from build123d import *

# Parameters (mm, degrees)
SKETCH_1_R          = 15
SKETCH_1_R_2        = 4.4
SKETCH_1_R_3        = 1.45
EXTRUDE_1_DEPTH     = 21
SKETCH_2_R          = 7.7
CUT_EXTRUDE_1_DEPTH = 4
SKETCH_3_R          = 11.25
CUT_EXTRUDE_2_DEPTH = 9.5
SKETCH_4_R          = 0.9
CUT_EXTRUDE_3_DEPTH = 4
SKETCH_5_W          = 6.5
SKETCH_5_H          = 9
CUT_EXTRUDE_4_DEPTH = 2


with BuildPart() as part:
    # 스케치1 → 보스-돌출1 (new body)
    with BuildSketch(Plane.XY):
        Circle(SKETCH_1_R)
        Circle(SKETCH_1_R_2, mode=Mode.SUBTRACT)
        with Locations((0, 6.25)):
            Circle(SKETCH_1_R_3, mode=Mode.SUBTRACT)
    extrude(amount=EXTRUDE_1_DEPTH)

    # 스케치2 → 컷-돌출1 (cut)
    with BuildSketch(Plane(origin=(0, 0, 0), x_dir=(-1, 0, 0), z_dir=(0, 0, -1))):
        Circle(SKETCH_2_R)
    extrude(amount=-CUT_EXTRUDE_1_DEPTH, mode=Mode.SUBTRACT)

    # 스케치3 → 컷-돌출2 (cut)
    with BuildSketch(Plane.XY.offset(21)):
        Circle(SKETCH_3_R)
    extrude(amount=-CUT_EXTRUDE_2_DEPTH, mode=Mode.SUBTRACT)

    # 스케치4 → 컷-돌출3 (cut)
    with BuildSketch(Plane.XY.offset(21)):
        with Locations((13, 0)):
            Circle(SKETCH_4_R)
        with Locations((6.5, -11.258330249)):
            Circle(SKETCH_4_R)
        with Locations((-6.5, -11.258330249)):
            Circle(SKETCH_4_R)
        with Locations((-13, 0)):
            Circle(SKETCH_4_R)
        with Locations((-6.5, 11.258330249)):
            Circle(SKETCH_4_R)
        with Locations((6.5, 11.258330249)):
            Circle(SKETCH_4_R)
    extrude(amount=-CUT_EXTRUDE_3_DEPTH, mode=Mode.SUBTRACT)

    # 스케치5 → 컷-돌출4 (cut)
    with BuildSketch(Plane.XY.offset(21)):
        with Locations((0, 12)):
            Rectangle(SKETCH_5_W, SKETCH_5_H)
    extrude(amount=-CUT_EXTRUDE_4_DEPTH, mode=Mode.SUBTRACT)


solid = part.part
CAD build for the part. Positions are in the model's coordinates, mm. A direction names the side the tool comes from. Give positions to 0.01 mm unless a question says otherwise; leave off trailing zeros. Write each loop counter-clockwise with the first axis right and the second up, starting at its lowest first coordinate (ties: lowest second). Pieces come first, ordered by that corner, then holes. Notation, with made-up numbers: (26.25, 52.25) - (70.25, 52.25) arc R17 ccw to (70.25, 71.25) - close; hole circle Ø8 at (-12.75, 46). An arc over 180 degrees is marked (long way). Put each result on its own line as item: value.
(1) Drop flat-ended pins along their axis: pin 1 Ø2 at (x, y) = (1, 13.5) entering from +Z; pin 2 Ø10 at (x, y) = (4.5, -4) entering from +Z; pin 3 Ø8 at (y, z) = (-7.5, 18.5) entering from +X. Give the stop position or say it passes through.
Working result:
pin 1: z = 19
pin 2: z = 11.5
pin 3: x = 14.59
(2) Saw through at D-D (z = 10.25). List the corners of the cut face in (x, y).
Working result:
outline: circle Ø30 at (0, 0); hole circle Ø8.8 at (0, 0); hole circle Ø2.9 at (0, 6.25)
(3) Saw through at A-A (y = 2.25). List the corners of the cut face in (x, z), then the cut area to 3 significant figures.
Working result:
outline: (-14.83, 0) - (-7.36, 0) - (-7.36, 4) - (-3.78, 4) - (-3.78, 11.5) - (-11.02, 11.5) - (-11.02, 21) - (-14.83, 21) - close; (3.78, 4) - (7.36, 4) - (7.36, 0) - (14.83, 0) - (14.83, 21) - (11.02, 21) - (11.02, 11.5) - (3.78, 11.5) - close
area: 298 mm^2
(4) Tool access for faces 1 (the flat face through (6, 11, 17)), 2 (the flat face through (3.25, 13, 20)), 3 (the cylindrical face through (-0.189, 7.688, 7.698)): list every direction of +Z, -Z, +X, -X, +Y, -Y with a clear straight run to the whole face (end or side of a thin tool).
Working result:
face 1: +Z
face 2: +Z, +Y
face 3: +Z, -Z
(5) Wall check: L1, parallel to Y at x = 6.5, z = 18.7; L2, parallel to Y at x = 0.75, z = 8.5; L3, parallel to X at y = 0, z = 9. Give the ranges that are in metal, low to high.
Working result:
L1: -13.52 to -12.16, -10.36 to -9.18, 9.18 to 10.36, 12.16 to 13.52
L2: -14.98 to -4.34, 4.34 to 5.01, 7.49 to 14.98
L3: -15 to -4.4, 4.4 to 15
(6) Pull direction Y, two halves, no side cores. Call faces 4 (the flat face through (-3.25, 13, 20)), 5 (the cylindrical face through (-6.62, 12.15, 19.03)), 6 (the cylindrical face through (-3.252, -14.643, 10.353)): released by +Y, released by -Y, zero draft, split by the parting line, or undercut.
Working result:
face 4: zero draft
face 5: undercut
face 6: split by the parting line
(7) Saw through at B-B (x = -1). List the corners of the cut face in (y, z), then the cut area to 3 significant figures.
Working result:
outline: (-14.97, 0) - (-7.63, 0) - (-7.63, 4) - (-4.28, 4) - (-4.28, 11.5) - (-11.21, 11.5) - (-11.21, 21) - (-14.97, 21) - close; (4.28, 4) - (5.2, 4) - (5.2, 11.5) - (4.28, 11.5) - close; (7.3, 4) - (7.63, 4) - (7.63, 0) - (14.97, 0) - (14.97, 19) - (11.21, 19) - (11.21, 11.5) - (7.3, 11.5) - close
area: 267 mm^2
(8) Saw through at C-C (x = -4). List the corners of the cut face in (y, z).
Working result:
outline: (-14.46, 0) - (-6.58, 0) - (-6.58, 4) - (-1.83, 4) - (-1.83, 11.5) - (-10.51, 11.5) - (-10.51, 21) - (-14.46, 21) - close; (1.83, 4) - (6.58, 4) - (6.58, 0) - (14.46, 0) - (14.46, 21) - (10.51, 21) - (10.51, 11.5) - (1.83, 11.5) - close
